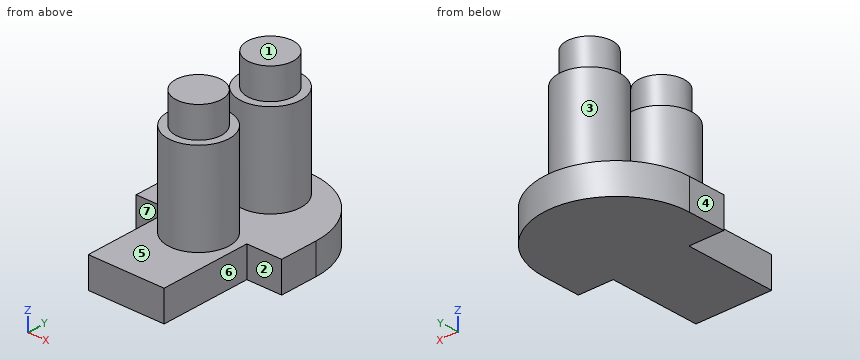
```python
from build123d import *

# Parameters (mm, degrees)
BOSS_EXTRUDE1_DEPTH = 4
SKETCH2_W           = 2.5
SKETCH2_H           = 4
CUT_EXTRUDE1_DEPTH  = 4
SKETCH4_R           = 4
BOSS_EXTRUDE2_DEPTH = 16
SKETCH5_R           = 3
BOSS_EXTRUDE3_DEPTH = 4


with BuildPart() as part:
    # Sketch1 → Boss-Extrude1 (new body)
    with BuildSketch(Plane.XY):
        with BuildLine():
            Line((0, 0), (10, 0))
            Line((10, 0), (10, 4))
            Line((10, 4), (12.5, 4))
            Line((12.5, 4), (12.5, 8))
            Line((12.5, 8), (10, 8))
            Line((10, 8), (10, 12))
            Line((10, 12), (14.6, 12))
            Line((14.6, 12), (14.6, 17))
            ThreePointArc((14.6, 17), (5, 26.6), (-4.6, 17))
            Line((-4.6, 17), (-4.6, 12))
            Line((-4.6, 12), (0, 12))
            Line((0, 12), (0, 8))
            Line((0, 8), (-2.5, 8))
            Line((-2.5, 8), (-2.5, 4))
            Line((-2.5, 4), (0, 4))
            Line((0, 4), (0, 0))
        make_face()
    extrude(amount=BOSS_EXTRUDE1_DEPTH)

    # Sketch2 → Cut-Extrude1 (cut)
    with BuildSketch(Plane.XY.offset(4)):
        with Locations((-1.25, 6)):
            Rectangle(SKETCH2_W, SKETCH2_H)
        with Locations((11.25, 6)):
            Rectangle(SKETCH2_W, SKETCH2_H)
    extrude(amount=-CUT_EXTRUDE1_DEPTH, mode=Mode.SUBTRACT)

    # Sketch4 → Boss-Extrude2 (add)
    with BuildSketch(Plane.XY):
        with Locations((5, 20.921172359)):
            Circle(SKETCH4_R)
        with Locations((5, 10.5)):
            Circle(SKETCH4_R)
    extrude(amount=BOSS_EXTRUDE2_DEPTH)

    # Sketch5 → Boss-Extrude3 (add)
    with BuildSketch(Plane.XY.offset(16)):
        with Locations((5, 10.5)):
            Circle(SKETCH5_R)
        with Locations((5, 20.921172359)):
            Circle(SKETCH5_R)
    extrude(amount=BOSS_EXTRUDE3_DEPTH)


solid = part.part
```
Read the model definition and answer for the solid it produces. Units are mm, in the model's axes. Face numbers are marked on the shaded views. A direction names the side the tool comes from. Coordinates: 2 decimals unless noted, no trailing zeros. Loops run counter-clockwise (first coordinate to the right, second up) from the corner with the lowest first, then second, coordinate; pieces in that order, holes last. Notation, with made-up numbers: (43, 36) -> (89, 36) arc R38 ccw to (89, 74) -> close; hole circle Ø4 at (69.25, 64.5). An arc over 180 degrees is marked (long way). Return JSON: item names as keys, results as strings.
Item 1: Find section C-C (z = 5.25). Determine the outline of the cut face in (x, y), plus the area to 3 significant figures.
Answers:
{"outline": "circle Ø8 at (5, 10.5); circle Ø8 at (5, 20.92)", "area": "101 mm2"}
Item 2: Find the intervals of material crossed by probe 1 along Z at (x, y) = (9.5, 11.25); probe 2 along X at (y, z) = (2.5, 1); probe 3 along Y at (x, z) = (7.75, 5.5), in increasing order.
Answers:
{"probe 1": "z = 0 to 4", "probe 2": "x = 0 to 10", "probe 3": "y = 7.6 to 13.4, 18.02 to 23.83"}
Item 3: Find section A-A (y = 10.5). Determine the outline of the cut face in (x, z), plus the area to 3 significant figures.
Answers:
{"outline": "(0, 0) -> (10, 0) -> (10, 4) -> (9, 4) -> (9, 16) -> (8, 16) -> (8, 20) -> (2, 20) -> (2, 16) -> (1, 16) -> (1, 4) -> (0, 4) -> close", "area": "160 mm2"}
Item 4: For a pull along Y with two mould halves and no side action, classify the marked faces 1, 2 and 3 as +Y half, -Y half, draft (parallel to the pull), parting line (faces both ways), or undercut.
Answers:
{"face 1": "draft", "face 2": "-Y half", "face 3": "undercut"}
Item 5: Find section B-B (x = 5). Determine the outline of the cut face in (y, z), plus the area to 3 significant figures.
Answers:
{"outline": "(0, 0) -> (26.6, 0) -> (26.6, 4) -> (24.92, 4) -> (24.92, 16) -> (23.92, 16) -> (23.92, 20) -> (17.92, 20) -> (17.92, 16) -> (16.92, 16) -> (16.92, 4) -> (14.5, 4) -> (14.5, 16) -> (13.5, 16) -> (13.5, 20) -> (7.5, 20) -> (7.5, 16) -> (6.5, 16) -> (6.5, 4) -> (0, 4) -> close", "area": "346 mm2"}
Item 6: Flat-ended cylindrical pins translate along their axes: P1, Ø3, axis at y = 8.5, z = 1, coming from the +X side; P2, Ø3, axis at y = 3.5, z = 2.5, coming from the -X side; P3, Ø1, axis at x = 11.5, y = 13, coming from the +Z side. Find the tip coordinate at first contact, or state that the pin passes through.
Answers:
{"P1": "stops at x = 10", "P2": "stops at x = 0", "P3": "stops at z = 4"}
Item 7: For the marked faces 4, 5, 6 and 7, determine the directions among +Z, -Z, +X, -X, +Y, -Y from which every point of the face is accessible in a straight line to the end or side of a thin tool.
Answers:
{"face 4": "+Z, -Z, -X, +Y, -Y", "face 5": "+Z", "face 6": "+Z, -Z, +X, -Y", "face 7": "+Z, -Z, -X, -Y"}
Item 8: Find section D-D (y = 22.5). Determine the outline of the cut face in (x, z).
Answers:
{"outline": "(-2.87, 0) -> (12.87, 0) -> (12.87, 4) -> (8.68, 4) -> (8.68, 16) -> (7.55, 16) -> (7.55, 20) -> (2.45, 20) -> (2.45, 16) -> (1.32, 16) -> (1.32, 4) -> (-2.87, 4) -> close"}
